Can you work these out from the model? Positions are in its coordinate system, mm. Face numbers are marked on the shaded views. A direction names the side the tool comes from. Round coordinates to 2 decimals unless told otherwise and drop trailing zeros. Order: outer loops, then holes, each group sorted by start corner. A loop starts at its lowest first (then second) coordinate and runs counter-clockwise, first axis right, second up.
Q1. For the marked faces 4, 5, 6 and 7, which set-ups out of +Z, -Z, +X, -X, +Y, -Y let a thin tool reach every point of the face, with its end or its side?
Q2. If we section it at B-B (x = 14.3): Please give me the cut outline in (y, z).
Q3. Will these pins go through, and if not, where does the flat tip stop? P1, Ø2.5, axis at x = 14.3, z = -3, coming from the -Y side; P2, Ø4.5, axis at y = 7, z = -8.5, coming from the -X side; P3, Ø5, axis at x = 14.3, z = -50.5, coming from the +Y side; P4, Ø3, axis at x = 38.5, y = 7, coming from the +Z side.
Q4. If we section it at A-A (y = 10.75): Please give me the cut outline in (x, z).
Q5. If I drill on line 1 (Z direction, x = 30, y = 5.5); line 2 (X direction, y = 5, z = -3); line 3 (X direction, y = 10.5, z = -42), over which ranges is the centre line in solid material (lowest first)?
Q6. We'd pull the mould along Z, two halves only. Please class the marked faces 1, 2 and 3: pulls with the +Z half, pulls with the -Z half, needs draft (parallel to the pull), parting line crosses it, or undercut.
Q7. If we section it at D-D (x = 36.5): Please give me the cut outline in (y, z), plus the area to 3 significant figures.
Q8. If we section it at C-C (z = -35): Please give me the cut outline in (x, y).
from build123d import *

# Parameters (mm, degrees)
SKETCH2_W           = 68.8
SKETCH2_H           = 53.5
BOSS_EXTRUDE1_DEPTH = 12.1
CUT_EXTRUDE1_DEPTH  = 12.1
SKETCH4_W           = 12.1
SKETCH4_H           = 10.6
BOSS_EXTRUDE2_DEPTH = 6.4
SKETCH5_W           = 9.1
SKETCH5_H           = 10.9
BOSS_EXTRUDE3_DEPTH = 1.8
SKETCH7_R           = 1.5
CUT_EXTRUDE2_DEPTH  = 12.1
SKETCH8_W           = 66.515944673
SKETCH8_H           = 48.513400954
CUT_EXTRUDE3_DEPTH  = 9.6


with BuildPart() as part:
    # Sketch2 → Boss-Extrude1 (new body)
    with BuildSketch(Plane(origin=(0, 0, 0), x_dir=(1, 0, 0), z_dir=(0, 1, 0))):
        with Locations((34.4, 26.75)):
            Rectangle(SKETCH2_W, SKETCH2_H)
    extrude(amount=BOSS_EXTRUDE1_DEPTH)

    # Sketch3 → Cut-Extrude1 (cut)
    with BuildSketch(Plane(origin=(0, 12.1, 0), x_dir=(1, 0, 0), z_dir=(0, 1, 0))):
        Polygon((68.8, 0), (68.8, 4.7), (66.6, 2.5), (66.6, 0), align=None)
        Polygon((68.8, 53.5), (66.6, 53.5), (66.6, 40.7), (68.8, 38.5), align=None)
    extrude(amount=-CUT_EXTRUDE1_DEPTH, mode=Mode.SUBTRACT)

    # Sketch4 → Boss-Extrude2 (add)
    with BuildSketch(Plane.ZY):
        with Locations((-38.85, 6.8)):
            Rectangle(SKETCH4_W, SKETCH4_H)
    extrude(amount=BOSS_EXTRUDE2_DEPTH)

    # Sketch5 → Boss-Extrude3 (add)
    with BuildSketch(Plane.ZY):
        with Locations((-8.15, 6.95)):
            Rectangle(SKETCH5_W, SKETCH5_H)
    extrude(amount=BOSS_EXTRUDE3_DEPTH)

    # Sketch7 → Cut-Extrude2 (cut)
    with BuildSketch(Plane(origin=(0, 12.1, 0), x_dir=(1, 0, 0), z_dir=(0, 1, 0))):
        with Locations(Location((14.3, 50.5, 0), (0, 0, 270))):
            Circle(SKETCH7_R)
        with Locations(Location((14.3, 3, 0), (0, 0, 270))):
            Circle(SKETCH7_R)
    extrude(amount=-CUT_EXTRUDE2_DEPTH, mode=Mode.SUBTRACT)

    # Sketch8 → Cut-Extrude3 (cut)
    with BuildSketch(Plane(origin=(0, 12.1, 0), x_dir=(1, 0, 0), z_dir=(0, 1, 0))):
        with Locations((50.682931162, 26.843299523)):
            Rectangle(SKETCH8_W, SKETCH8_H)
    extrude(amount=-CUT_EXTRUDE3_DEPTH, mode=Mode.SUBTRACT)


solid = part.part
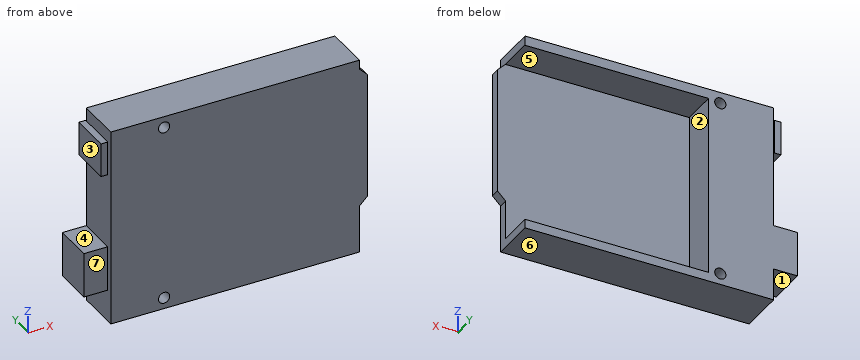
Solution:
1. face 4: -X, +Y, -Y
1. face 5: +X, +Y
1. face 6: -Z, +X, -X, +Y, -Y
1. face 7: +Z, -Z, -X, -Y
2. outline: (0, -53.5) - (12.1, -53.5) - (12.1, -52) - (0, -52) - close; (0, -49) - (12.1, -49) - (12.1, -4.5) - (0, -4.5) - close; (0, -1.5) - (12.1, -1.5) - (12.1, 0) - (0, 0) - close
3. P1: passes through
3. P2: stops at x = -1.8
3. P3: stops at y = 12.1
3. P4: stops at z = 0
4. outline: (-6.4, -44.9) - (0, -44.9) - (0, -53.5) - (66.6, -53.5) - (66.6, -51.1) - (17.42, -51.1) - (17.42, -2.59) - (66.69, -2.59) - (66.6, -2.5) - (66.6, 0) - (0, 0) - (0, -3.6) - (-1.8, -3.6) - (-1.8, -12.7) - (0, -12.7) - (0, -32.8) - (-6.4, -32.8) - close; hole circle Ø3 at (14.3, -50.5); hole circle Ø3 at (14.3, -3)
5. line 1: z = -53.5 to -51.1, -2.59 to 0
5. line 2: x = 0 to 12.8, 15.8 to 17.42
5. line 3: x = -6.4 to 17.42
6. face 1: pulls with the -Z half
6. face 2: undercut
6. face 3: needs draft
7. outline: (0, -53.5) - (12.1, -53.5) - (12.1, -51.1) - (2.5, -51.1) - (2.5, -2.59) - (12.1, -2.59) - (12.1, 0) - (0, 0) - close
7. area: 182 mm2
8. outline: (-6.4, 1.5) - (0, 1.5) - (0, 0) - (68.8, 0) - (68.8, 2.5) - (17.42, 2.5) - (17.42, 12.1) - (-6.4, 12.1) - close
